Can you work these out from the model? Positions are in its coordinate system, mm. A direction names the side the tool comes from. Round coordinates to 2 decimals unless told otherwise and drop trailing zeros. Order: outer loops, then holes, each group sorted by start corner. A loop starts at its lowest first (then second) coordinate and runs counter-clockwise, first axis right, second up. Notation, with made-up numbers: (3, -1) -> (8, -1) arc R27 ccw to (8, 29) -> close; hole circle Ø8 at (52, -39). An arc over 180 degrees is marked (long way). Use a Markdown table: item, result. Add a question column.
Q1. For faces 4 (the face through (210, 2, -135)), 5 (the face through (13.5, 2, -123)), which set-ups out of +Z, -Z, +X, -X, +Y, -Y let a thin tool reach every point of the face, with its end or its side?
Q2. If we section it at A-A on z = -67: List the corners of the cut face in (x, y) for me.
Q3. I need wall thicknesses on line 1 along X through (y, z) = (1.9, -80); line 2 along X through (y, z) = (2.25, -115); line 3 along Z through (x, y) = (20, 3.8). Which ranges of each line are inside material? Lowest first, please. Write a range as [from, to].
Q4. We'd pull the mould along X, two halves only. Please class faces 1 (the face through (205, 2, -80)), 2 (the face through (143.5, 2, -37)), 3 (the face through (207, 2, -50)): +X half, -X half, draft (parallel to the pull), parting line (faces both ways), or undercut.
Q5. If we section it at B-B on y = 2: Give the number of separate pieces and of enclosed holes in the cut face, plus the area to 3 significant figures.
Autodesk Inventor part; units mm, degrees
ref_plane "YZ Plane" through (0, 0, 0) normal (1, 0, 0) x (0, 1, 0)
ref_plane "XZ Plane" through (0, 0, 0) normal (0, 1, 0) x (-1, 0, 0)
ref_plane "XY Plane" through (0, 0, 0) normal (0, 0, 1) x (1, 0, 0)
sketch "Sketch1" plane through (0, 0, 0) normal (0, 1, 0) x (-1, 0, 0)
  line L0 (0, 0) -> (-210, 0)
  line L1 (-210, 0) -> (-210, -160)
  line L2 (-210, -160) -> (0, -160)
  line L3 (75, -80) -> (-210, -80) construction
  line L4 (-105, 0) -> (-105, -160) construction
  line L5 (-40, 0) -> (-40, -160) construction
  line L6 (-133, 0) -> (-133, -160) construction
  line L7 (-15, -130) -> (-15, -115) construction
  line L8 (-15, -130) -> (-15, -115) construction
  line L9 (-13.5, -130) -> (-13.5, -115)
  line L10 (-16.5, -115) -> (-16.5, -130)
  arc A0 (-16.5, -130) -> (-13.5, -130) centre (-15, -130) ccw
  arc A1 (-13.5, -115) -> (-16.5, -115) centre (-15, -115) ccw
  line L11 (-65, -130) -> (-65, -115) construction
  line L12 (-65, -130) -> (-65, -115) construction
  line L13 (-66.5, -130) -> (-66.5, -115)
  line L14 (-63.5, -115) -> (-63.5, -130)
  arc A2 (-66.5, -130) -> (-63.5, -130) centre (-65, -130) ccw
  arc A3 (-63.5, -115) -> (-66.5, -115) centre (-65, -115) ccw
  line L15 (-125, -160) -> (-85, -160)
  line L16 (-85, -160) -> (-85, -155)
  line L17 (-85, -155) -> (-125, -155)
  line L18 (-125, -155) -> (-125, -160)
  line L19 (-195, -130) -> (-195, -115) construction
  line L20 (-195, -130) -> (-195, -115) construction
  line L21 (-196.5, -130) -> (-196.5, -115)
  line L22 (-193.5, -115) -> (-193.5, -130)
  arc A4 (-196.5, -130) -> (-193.5, -130) centre (-195, -130) ccw
  arc A5 (-193.5, -115) -> (-196.5, -115) centre (-195, -115) ccw
  line L23 (-146.5, -115) -> (-146.5, -130)
  line L24 (-145, -130) -> (-145, -115) construction
  line L25 (-143.5, -130) -> (-143.5, -115)
  arc A6 (-146.5, -130) -> (-143.5, -130) centre (-145, -130) ccw
  line L26 (-145, -130) -> (-145, -115) construction
  arc A7 (-143.5, -115) -> (-146.5, -115) centre (-145, -115) ccw
  line L27 (-105, -160) -> (-105, 0) construction
  line L28 (-15, -30) -> (-15, -45) construction
  line L29 (-15, -30) -> (-15, -45) construction
  line L30 (-13.5, -30) -> (-13.5, -45)
  line L31 (-16.5, -45) -> (-16.5, -30)
  arc A8 (-13.5, -30) -> (-16.5, -30) centre (-15, -30) ccw
  arc A9 (-16.5, -45) -> (-13.5, -45) centre (-15, -45) ccw
  line L32 (-63.5, -45) -> (-63.5, -30)
  line L33 (-65, -30) -> (-65, -45) construction
  line L34 (-66.5, -30) -> (-66.5, -45)
  arc A10 (-63.5, -30) -> (-66.5, -30) centre (-65, -30) ccw
  line L35 (-65, -30) -> (-65, -45) construction
  arc A11 (-66.5, -45) -> (-63.5, -45) centre (-65, -45) ccw
  line L36 (-125, 0) -> (-85, 0)
  line L37 (-85, 0) -> (-85, -5)
  line L38 (-85, -5) -> (-125, -5)
  line L39 (-125, -5) -> (-125, 0)
  arc A12 (-193.5, -30) -> (-196.5, -30) centre (-195, -30) ccw
  line L40 (-193.5, -45) -> (-193.5, -30)
  line L41 (-195, -30) -> (-195, -45) construction
  line L42 (-195, -30) -> (-195, -45) construction
  arc A13 (-196.5, -45) -> (-193.5, -45) centre (-195, -45) ccw
  line L43 (-196.5, -30) -> (-196.5, -45)
  line L44 (-146.5, -45) -> (-146.5, -30)
  line L45 (-145, -30) -> (-145, -45) construction
  line L46 (-145, -30) -> (-145, -45) construction
  arc A14 (-146.5, -45) -> (-143.5, -45) centre (-145, -45) ccw
  line L47 (-143.5, -30) -> (-143.5, -45)
  arc A15 (-143.5, -30) -> (-146.5, -30) centre (-145, -30) ccw
  line L48 (-210, -12.5) -> (-210, -62.5)
  line L49 (-210, -62.5) -> (-210, -110)
  line L50 (-210, -110) -> (-205, -110)
  line L51 (-205, -110) -> (-205, -50)
  line L52 (-205, -50) -> (-210, -50)
  line L53 (-210, -50) -> (-210, -12.5)
  line L54 (0, -160) -> (0, 0)
  point P0 (-15, -122.5)
  point P1 (-65, -122.5)
  point P2 (-195, -122.5)
  point P3 (-145, -122.5)
  point P4 (-15, -37.5)
  point P5 (-65, -37.5)
  point P6 (-195, -37.5)
  point P7 (-145, -37.5)
  point P8 (-65, -122.5)
  point P9 (-15, -122.5)
  point P10 (-125, -160)
  point P11 (-85, -160)
  point P12 (-85, 0)
  point P13 (-125, 0)
  point P14 (-195, -122.5)
  dimension "d2" = 15
  dimension "d4" = 30
  dimension "d6" = 1.5
  dimension "d9" = 40
  dimension "d13" = 0
  dimension "d14" = 5
  dimension "d16" = 20
  dimension "d22" = 5
  dimension "d26" = 30
  dimension "d27" = 30
  dimension "d28" = 0
  dimension "d30" = 160
  dimension "d32" = 50
  dimension "d56" = 15
  dimension "d57" = 210
extrude "Extrusion1" add sketch "Sketch1" along normal blind 5 contours L54 L2 L16 L17 L18 L1 L50 L51 L52 L0 L39 L38 L37 | L37 L38 L39 L0 | L2 L18 L17 L16
sketch "Sketch4" plane through (0, 5, 0) normal (0, 1, 0) x (1, 0, 0)
  line L0 (0, 0) -> (210, 0)
  line L1 (0, 160) -> (0, 0)
  point P0 (20, 80)
  dimension "d76" = 80
  dimension "d77" = 20
hole "Hole3" at (20, 5, -80) direction (0, -1, 0) diameter 3 end through all
sketch "Sketch5" plane through (0, 5, 0) normal (0, 1, 0) x (1, 0, 0)
  line L0 (205, 50) -> (205, 110)
  point P0 (0, 0)
  point P1 (190, 80)
  dimension "d85" = 15
  dimension "d86" = 30
hole "Hole4" at (190, 5, -80) direction (0, -1, 0) diameter 3 end through all
properties part number "base_2" material "Acrylic"
Answer below:
| question | item | result |
|---|---|---|
| 1 | face 4 | +Z, -Z, +X, +Y, -Y |
| 1 | face 5 | +Y, -Y |
| 2 | outline | (0, 0) -> (205, 0) -> (205, 5) -> (0, 5) -> close |
| 3 | line 1 | [0, 18.5], [21.5, 188.5], [191.5, 205] |
| 3 | line 2 | [0, 13.5], [16.5, 63.5], [66.5, 143.5], [146.5, 193.5], [196.5, 210] |
| 3 | line 3 | [-160, -81.5], [-78.5, 0] |
| 4 | face 1 | +X half |
| 4 | face 2 | undercut |
| 4 | face 3 | draft |
| 5 | separate pieces | 1 |
| 5 | enclosed holes | 10 |
| 5 | area | 32,900 mm² |
